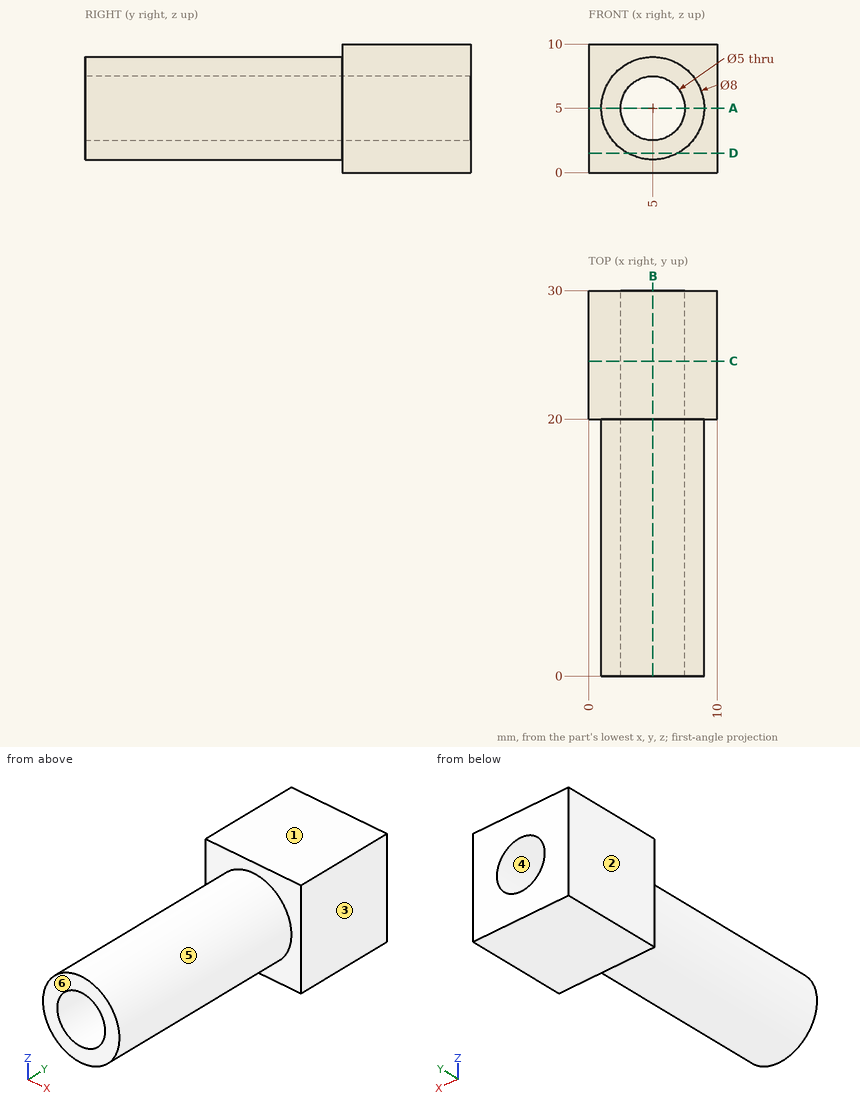
Part print with two shaded views. Sizes in mm from the minimum x, y, z corner. A direction names the side the tool comes from. Coordinates: 2 decimals unless noted, no trailing zeros. Order: outer loops, then holes, each group sorted by start corner. A loop starts at its lowest first (then second) coordinate and runs counter-clockwise, first axis right, second up. Notation, with made-up numbers: M -34,45 L -9,45 A10 cw -9,57 Z; hole C 28,69 d11. An arc over 180 degrees is marked long. Use a Markdown table: item, result.
(1) Tool access for the marked faces 5 and 6: list every direction of +Z, -Z, +X, -X, +Y, -Y with a clear straight run to the whole face (end or side of a thin tool).
A:
| item | result |
|---|---|
| face 5 | -Y |
| face 6 | +Z, -Z, +X, -X, -Y |
(2) Flat gauge pins, fed straight in: pin 1 (1 mm diameter, centred on y = 5.5, z = 1.5, fed in from -X); pin 2 (1.5 mm diameter, centred on y = 11.5, z = 2, fed in from +X). Where does each tip first touch, or does it go through?
A:
| item | result |
|---|---|
| pin 1 | stops at x = 2.35 |
| pin 2 | stops at x = 8.31 |
(3) Cut at B-B on x = 5. Write the cut outline in (y, z).
A:
| item | result |
|---|---|
| outline | M 0,1 L 20,1 L 20,0 L 30,0 L 30,2.5 L 0,2.5 Z; M 0,7.5 L 30,7.5 L 30,10 L 20,10 L 20,9 L 0,9 Z |
(4) Cut at D-D on z = 1.5. Write the cut outline in (x, y).
A:
| item | result |
|---|---|
| outline | M 0,20 L 3.06,20 L 3.06,0 L 6.94,0 L 6.94,20 L 10,20 L 10,30 L 0,30 Z |
(5) Probe L1, parallel to X at y = 24, z = 5; L2, parallel to X at y = 13.25, z = 5; L3, parallel to Y at x = 8.75, z = 6.5. List the from-to ranges inside material, lowest first.
A:
| item | result |
|---|---|
| L1 | x = 0 to 2.5, 7.5 to 10 |
| L2 | x = 1 to 2.5, 7.5 to 9 |
| L3 | y = 20 to 30 |
(6) Cut at C-C on y = 24.5. Write the cut outline in (x, z).
A:
| item | result |
|---|---|
| outline | M 0,0 L 10,0 L 10,10 L 0,10 Z; hole C 5,5 d5 |
(7) Pull direction X, two halves, no side cores. Call the marked faces 1, 2, 3 and 4: released by +X, released by -X, zero draft, split by the parting line, or undercut.
A:
| item | result |
|---|---|
| face 1 | zero draft |
| face 2 | released by -X |
| face 3 | released by +X |
| face 4 | undercut |
(8) Cut at A-A on z = 5. Write the cut outline in (x, y).
A:
| item | result |
|---|---|
| outline | M 0,20 L 1,20 L 1,0 L 2.5,0 L 2.5,30 L 0,30 Z; M 7.5,0 L 9,0 L 9,20 L 10,20 L 10,30 L 7.5,30 Z |
